Design review of the part built by this model. Coordinates are the model's own, in mm. A direction names the side the tool comes from. Coordinates: 2 decimals unless noted, no trailing zeros. Write each loop counter-clockwise with the first axis right and the second up, starting at its lowest first coordinate (ties: lowest second). Pieces come first, ordered by that corner, then holes. Notation, with made-up numbers: (-36.5, 82.25) - (13.5, 82.25) arc R23 ccw to (13.5, 115.25) - close; hole circle Ø8 at (42, 7.25). An arc over 180 degrees is marked (long way). Answer as CSV lines item,"result". Start each with the question number.
Q1. Clearance check with flat-ended pins moving along their axes: pin 1 (3 mm diameter, centred on x = 8, y = 0.5, fed in from -Z); pin 2 (1 mm diameter, centred on x = -1.5, z = 1, fed in from +Y); pin 3 (1.5 mm diameter, centred on y = -1, z = 3.5, fed in from +X). State where each tip first meets the part, or that it passes through.
Q2. We need section D-D (y = 0.25). State how many separate pieces and enclosed holes the cut face has, plus the area to 3 significant figures.
Q3. Mouldability with a two-part tool opening along Y and no side actions: class faces 1 (the face through (1, -1, 2)), 2 (the face through (15.95, -0.04, 3.14)), 3 (the face through (2, -2, 0)) as pulls with the +Y half, pulls with the -Y half, needs draft (parallel to the pull), parting line crosses it, or undercut.
Q4. We need section C-C (x = 14). Write out the cut boundary in (y, z), plus the area to 3 significant figures.
Q5. We need section B-B (z = 2.6). Write out the cut boundary in (x, y).
Q6. We need section A-A (x = 0). Write out the cut boundary in (y, z), plus the area to 3 significant figures.
Q7. Machinability: for faces 4 (the face through (6, 1, 3.9)), 5 (the face through (-1.5, 0.07, 3.41)), 6 (the face through (-3.497, 0.154, 1.923)), which of the approach directions +Z, -Z, +X, -X, +Y, -Y give a long, thin tool a straight path to every point of the face, cutting with its end or side? Answer none if there is none.
Q8. For line 1 along Z through (x, y) = (11.5, -1.5); line 2 along Y through (x, z) = (8.32, 2.95); line 3 along Y through (x, z) = (6, 2.8), list the stretches that pass through material, from the lowest coordinate up. Write a range as [from, to].
from build123d import *

# Parameters (mm, degrees)
SKETCH_1_R          = 3.5
EXTRUDE_1_DEPTH     = 3.9
EXTRUDE_START       = 2.4
SKETCH_1_6_R        = 0.6
EXTRUDE_2_DEPTH     = 1.5
SKETCH_1_3_R        = 2.5
CUT_EXTRUDE_1_DEPTH = 2
CUT_EXTRUDE_START   = 3.9
SKETCH_1_4_R        = 1.5
CUT_EXTRUDE_2_DEPTH = 1
SKETCH_1_5_R        = 1
CUT_EXTRUDE_3_DEPTH = 17.788761122


with BuildPart() as part:
    # 草图1 → 凸台-拉伸1 (new body)
    with BuildSketch(Plane.XY):
        Circle(SKETCH_1_R)
    extrude(amount=EXTRUDE_1_DEPTH)

    # 草图1<6> → 凸台-拉伸2 (add)
    with BuildSketch(Plane.XY.offset(EXTRUDE_START)):
        with BuildLine():
            Line((14.170277633, 1.89618915), (2.286372673, 2.65))
            ThreePointArc((2.286372673, 2.65), (3.5, 0), (2.286372673, -2.65))
            Line((2.286372673, -2.65), (14.170277633, -1.89618915))
            ThreePointArc((14.170277633, -1.89618915), (15.95, 0), (14.170277633, 1.89618915))
        make_face()
        with BuildLine():
            ThreePointArc((11.54, 0), (12.14, 0.6), (12.74, 0))
            ThreePointArc((12.74, 0), (12.14, -0.6), (11.54, 0))
        make_face(mode=Mode.SUBTRACT)
        with Locations((4.5, 0)):
            Circle(SKETCH_1_6_R, mode=Mode.SUBTRACT)
        with BuildLine():
            ThreePointArc((5.81, 0), (6.41, 0.6), (7.01, 0))
            ThreePointArc((7.01, 0), (6.41, -0.6), (5.81, 0))
        make_face(mode=Mode.SUBTRACT)
        with BuildLine():
            ThreePointArc((7.72, 0), (8.32, 0.6), (8.92, 0))
            ThreePointArc((8.92, 0), (8.32, -0.6), (7.72, 0))
        make_face(mode=Mode.SUBTRACT)
        with BuildLine():
            ThreePointArc((9.63, 0), (10.23, 0.6), (10.83, 0))
            ThreePointArc((10.83, 0), (10.23, -0.6), (9.63, 0))
        make_face(mode=Mode.SUBTRACT)
        with Locations((14.05, 0)):
            Circle(SKETCH_1_6_R, mode=Mode.SUBTRACT)
    extrude(amount=EXTRUDE_2_DEPTH)

    # 草图1<3> → 切除-拉伸1 (cut)
    with BuildSketch(Plane.XY):
        Circle(SKETCH_1_3_R)
    extrude(amount=CUT_EXTRUDE_1_DEPTH, mode=Mode.SUBTRACT)

    # 草图1<4> → 切除-拉伸2 (cut)
    with BuildSketch(Plane.XY.offset(CUT_EXTRUDE_START)):
        Circle(SKETCH_1_4_R)
    extrude(amount=-CUT_EXTRUDE_2_DEPTH, mode=Mode.SUBTRACT)

    # 草图1<5> → 切除-拉伸3 (cut, through all)
    with BuildSketch(Plane.XY):
        Circle(SKETCH_1_5_R)
    extrude(amount=CUT_EXTRUDE_3_DEPTH, mode=Mode.SUBTRACT)


solid = part.part
Results list:
1,pin 1,"stops at z = 2.4"
1,pin 2,"stops at y = 3.35"
1,pin 3,"stops at x = 15.93"
2,separate pieces,"8"
2,enclosed holes,"0"
2,area,"21.4 mm2"
3,face 1,"undercut"
3,face 2,"parting line crosses it"
3,face 3,"needs draft"
4,outline,"(-1.91, 2.4) - (-0.6, 2.4) - (-0.6, 3.9) - (-1.91, 3.9) - close; (0.6, 2.4) - (1.91, 2.4) - (1.91, 3.9) - (0.6, 3.9) - close"
4,area,"3.93 mm2"
5,outline,"(2.29, -2.65) - (14.17, -1.9) arc R1.9 ccw to (14.17, 1.9) - (2.29, 2.65) arc R3.5 ccw (long way) to start; hole circle Ø2 at (0, 0); hole circle Ø1.2 at (4.5, 0); hole circle Ø1.2 at (6.41, 0); hole circle Ø1.2 at (8.32, 0); hole circle Ø1.2 at (10.23, 0); hole circle Ø1.2 at (12.14, 0); hole circle Ø1.2 at (14.05, 0)"
6,outline,"(-3.5, 0) - (-2.5, 0) - (-2.5, 2) - (-1, 2) - (-1, 2.9) - (-1.5, 2.9) - (-1.5, 3.9) - (-3.5, 3.9) - close; (1, 2) - (2.5, 2) - (2.5, 0) - (3.5, 0) - (3.5, 3.9) - (1.5, 3.9) - (1.5, 2.9) - (1, 2.9) - close"
6,area,"12.5 mm2"
7,face 4,"+Z, +X, -X, +Y, -Y"
7,face 5,"+Z"
7,face 6,"-Z"
8,line 1,"z = [2.4, 3.9]"
8,line 2,"y = [-2.27, -0.6], [0.6, 2.27]"
8,line 3,"y = [-2.41, -0.44], [0.44, 2.41]"
